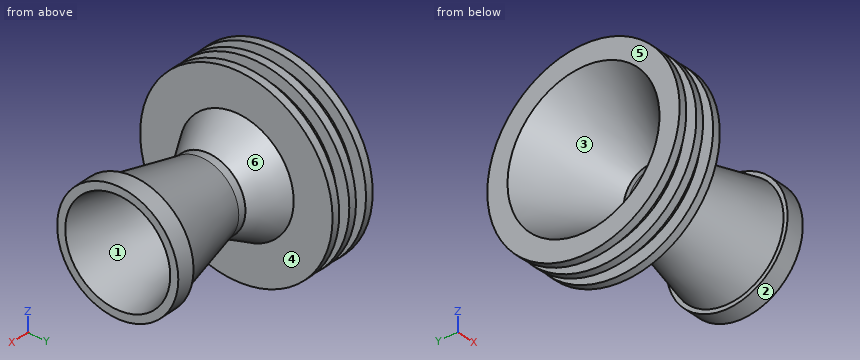
```python
from build123d import *


with BuildPart() as part:
    # Esboço2 → Revolução1 (revolve)
    with BuildSketch(Plane.XY):
        Polygon((0, 23.8125), (2, 23.8125), (2, 20.8125), (5, 20.8125), (5, 23.8125), (7, 23.8125), (7, 20.8125), (10, 20.8125), (10, 23.8125), (12, 23.8125), (12, 20.8125), (12, 14.193697846), (20.49192648, 9.290881808), (22.49192648, 9.290881808), (42.889358319, 14), (42.889358319, 15), (47.44870541, 15), (47.44870541, 13), (21.459850164, 7), (20.459850164, 7), (0, 18.8125), (0, 20.8125), align=None)
    revolve(axis=Axis((-1000, 0, 0), (1, 0, 0)))


solid = part.part
```
Can you work these out from the model? Positions are in its coordinate system, mm. Face numbers are marked on the shaded views. A direction names the side the tool comes from. Round coordinates to 2 decimals unless told otherwise and drop trailing zeros. Order: outer loops, then holes, each group sorted by start corner. A loop starts at its lowest first (then second) coordinate and runs counter-clockwise, first axis right, second up.
(1) If we section it at A-A (x = 41): Please give me the cut outline in (y, z).
Results are:
outline: circle Ø27.13 at (0, 0); hole circle Ø23.02 at (0, 0)
(2) If I drill on L1, parallel to Z at x = 21.1, y = 0; L2, parallel to X at y = -20.5, z = 6.5; L3, parallel to Z at x = 44.5, y = 1, over which ranges is the centre line in solid material (lowest first)?
Results are:
L1: z = -9.29 to -7, 7 to 9.29
L2: x = 0 to 2, 5 to 7, 10 to 12
L3: z = -14.97 to -12.28, 12.28 to 14.97
(3) On a 3-axis mill with a long thin cutter (end or side, diameter ignored), from which of +Z, -Z, +X, -X, +Y, -Y can I reach the whole of each face in a straight line? I mean the marked faces 5 and 6. Say none if no direction works.
Results are:
face 5: +Z, -Z, -X, +Y, -Y
face 6: none
(4) We'd pull the mould along Y, two halves only. Please class the marked faces 1, 2, 3 and 4: +Y half, -Y half, draft (parallel to the pull), parting line (faces both ways), or undercut.
Results are:
face 1: undercut
face 2: parting line
face 3: undercut
face 4: draft
(5) I'm going to push flat-ended pins straight in: pin 1 (12 mm diameter, centred on x = 34.5, z = 15, fed in from -Y); pin 2 (24 mm diameter, centred on y = -2, z = 4.5, fed in from -X); pin 3 (4 mm diameter, centred on x = 7.5, y = 3, fed in from +Z); pin 4 (6 mm diameter, centred on y = 7.5, z = -8.5, fed in from +X). Where does each tip first touch, or does it pass through?
Results are:
pin 1: stops at y = -8.35
pin 2: stops at x = 3.27
pin 3: stops at z = 23.79
pin 4: stops at x = 47.45
(6) If we section it at B-B (x = 14): Please give me the cut outline in (y, z), plus the area to 3 significant figures.
Results are:
outline: circle Ø26.08 at (0, 0); hole circle Ø21.46 at (0, 0)
area: 172 mm2
